Here's how the part is built. I have some questions about the finished solid (model axes, mm). Round coordinates to 2 decimals unless told otherwise and drop trailing zeros. Order: outer loops, then holes, each group sorted by start corner. A loop starts at its lowest first (then second) coordinate and runs counter-clockwise, first axis right, second up. Notation, with made-up numbers: (-0.5, 56.25) -> (35.5, 56.25) arc R11 ccw to (35.5, 62.25) -> close; hole circle Ø7 at (-30, 20.5). An arc over 180 degrees is marked (long way). Answer in a Markdown table with one row per item.
```python
from build123d import *

# Parameters (mm, degrees)
SKETCH1_W           = 340
SKETCH1_H           = 200
SKETCH1_R           = 3
SKETCH1_R_2         = 4.5
BOSS_EXTRUDE1_DEPTH = 5


with BuildPart() as part:
    # Sketch1 → Boss-Extrude1 (new body)
    with BuildSketch(Plane(origin=(0, 0, 0), x_dir=(1, 0, 0), z_dir=(0, 1, 0))):
        Rectangle(SKETCH1_W, SKETCH1_H)
        with Locations((155, 85)):
            Circle(SKETCH1_R, mode=Mode.SUBTRACT)
        with Locations((-155, 85)):
            Circle(SKETCH1_R, mode=Mode.SUBTRACT)
        with Locations((-155, -85)):
            Circle(SKETCH1_R, mode=Mode.SUBTRACT)
        with Locations((155, -85)):
            Circle(SKETCH1_R, mode=Mode.SUBTRACT)
        with Locations((0, 80)):
            Circle(SKETCH1_R_2, mode=Mode.SUBTRACT)
        with Locations((0, -80)):
            Circle(SKETCH1_R_2, mode=Mode.SUBTRACT)
        with Locations((90, 80)):
            Circle(SKETCH1_R_2, mode=Mode.SUBTRACT)
        with Locations((90, -80)):
            Circle(SKETCH1_R_2, mode=Mode.SUBTRACT)
        with Locations((-90, -80)):
            Circle(SKETCH1_R_2, mode=Mode.SUBTRACT)
        with Locations((-90, 80)):
            Circle(SKETCH1_R_2, mode=Mode.SUBTRACT)
    extrude(amount=BOSS_EXTRUDE1_DEPTH)


solid = part.part
```
1. Please list where these lines run through material, in increasing order: line 1 along Z through (x, y) = (90, 3.3); line 2 along X through (y, z) = (1.6, -85); line 3 along X through (y, z) = (2.4, -80).
Numbers:
| item | result |
|---|---|
| line 1 | z = -100 to -84.5, -75.5 to 75.5, 84.5 to 100 |
| line 2 | x = -170 to -158, -152 to 152, 158 to 170 |
| line 3 | x = -170 to -94.5, -85.5 to -4.5, 4.5 to 85.5, 94.5 to 170 |
2. Suppose I cut it at A-A on x = 90. Write out the boundary of the cut face in (y, z).
Numbers:
| item | result |
|---|---|
| outline | (0, -100) -> (5, -100) -> (5, -84.5) -> (0, -84.5) -> close; (0, -75.5) -> (5, -75.5) -> (5, 75.5) -> (0, 75.5) -> close; (0, 84.5) -> (5, 84.5) -> (5, 100) -> (0, 100) -> close |
3. We'd pull the mould along Z, two halves only. Please class faces 1 (the face through (-2, 5, -1)), 2 (the face through (-153.616, 2.465, -82.338)): released by +Z, released by -Z, zero draft, split by the parting line, or undercut.
Numbers:
| item | result |
|---|---|
| face 1 | zero draft |
| face 2 | undercut |
